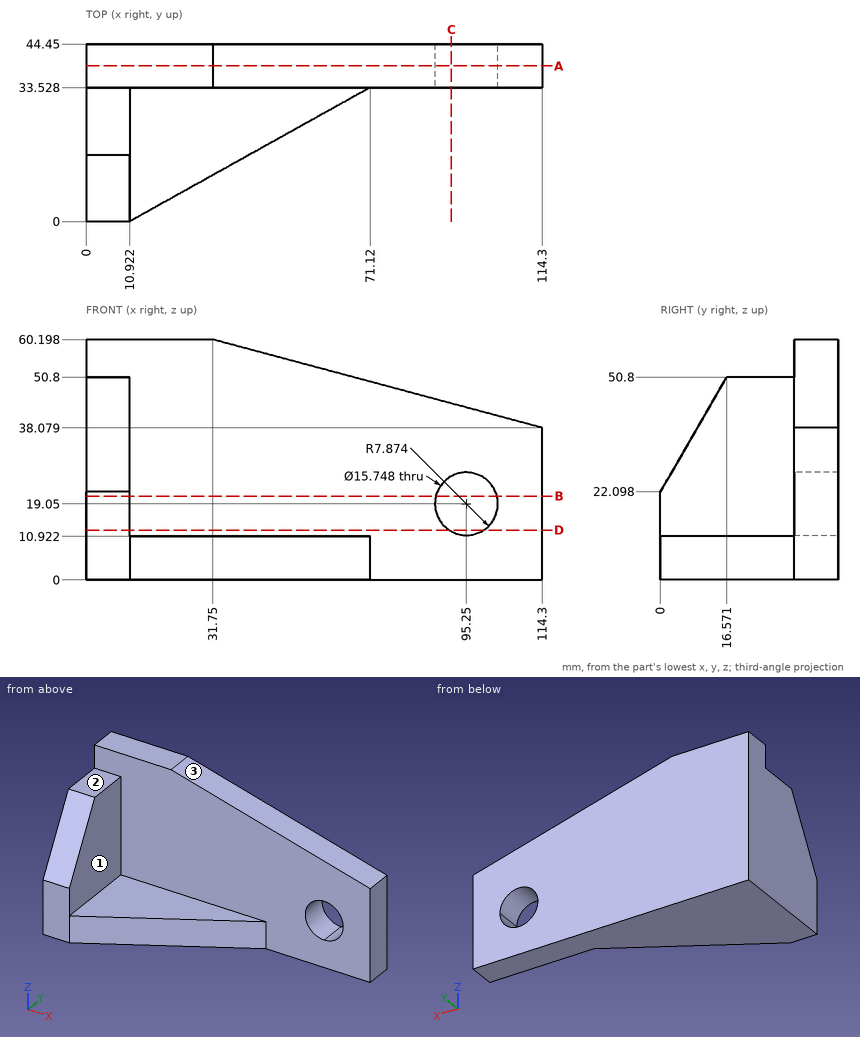
Can you work these out from the drawing? Everything is in mm from the part's minimum corner. A direction names the side the tool comes from. Round coordinates to 2 decimals unless told otherwise and drop trailing zeros. Loops run counter-clockwise (first coordinate to the right, second up) from the corner with the lowest first, then second, coordinate; pieces in that order, holes last. Notation, with made-up numbers: (11.5, 49) - (15.5, 49) arc R9 cw to (15.5, 65) - close; hole circle Ø5 at (14.5, -10). An arc over 180 degrees is marked (long way). Answer as CSV lines item,"result".
1. I want a section at B-B on z = 21. List the corners of the cut face in (x, y) for me, then the cut area to 3 significant figures.
Filled in:
outline,"(0, 0) - (10.92, 0) - (10.92, 33.53) - (87.62, 33.53) - (87.62, 44.45) - (0, 44.45) - close; (102.88, 33.53) - (114.3, 33.53) - (114.3, 44.45) - (102.88, 44.45) - close"
area,"1,450 mm^2"
2. For pin 1 Ø12 at (x, z) = (16.5, 36) entering from -Y; pin 2 Ø8.5 at (x, y) = (5.5, 22.5) entering from +Z; pin 3 Ø9.5 at (x, z) = (95.25, 19.05) entering from -Y, each with a flat end and sliding along its axis, tell me the tip position at first contact or that it passes through.
Filled in:
pin 1,"stops at y = 6.75"
pin 2,"stops at z = 50.8"
pin 3,"passes through"
3. I want a section at A-A on y = 39. List the corners of the cut face in (x, z) for me, then the cut area to 3 significant figures.
Filled in:
outline,"(0, 0) - (114.3, 0) - (114.3, 38.08) - (31.75, 60.2) - (0, 60.2) - close; hole circle Ø15.75 at (95.25, 19.05)"
area,"5,770 mm^2"
4. On a 3-axis mill with a long thin cutter (end or side, diameter ignored), from which of +Z, -Z, +X, -X, +Y, -Y can I reach the whole of each face in a straight line? I mean the marked faces 1, 2 and 3. Say none if no direction works.
Filled in:
face 1,"+Z, +X, -Y"
face 2,"+Z, +X, -X, -Y"
face 3,"+Z, +X, +Y, -Y"
5. I want a section at C-C on x = 91.5. List the corners of the cut face in (y, z) for me, then the cut area to 3 significant figures.
Filled in:
outline,"(33.53, 0) - (44.45, 0) - (44.45, 12.13) - (33.53, 12.13) - close; (33.53, 25.97) - (44.45, 25.97) - (44.45, 44.19) - (33.53, 44.19) - close"
area,"331 mm^2"
6. I want a section at D-D on z = 12.5. List the corners of the cut face in (x, y) for me.
Filled in:
outline,"(0, 0) - (10.92, 0) - (10.92, 33.53) - (90.88, 33.53) - (90.88, 44.45) - (0, 44.45) - close; (99.62, 33.53) - (114.3, 33.53) - (114.3, 44.45) - (99.62, 44.45) - close"
7. Please list where these lines run through material, in increasing order: line 1 along X through (y, z) = (42, 19.05); line 2 along Y through (x, z) = (96, 10); line 3 along Z through (x, y) = (8, 28). Write a range as [from, to].
Filled in:
line 1,"x = [0, 87.38], [103.12, 114.3]"
line 2,"y = [33.53, 44.45]"
line 3,"z = [0, 50.8]"
